from build123d import *

# Parameters (mm, degrees)
F0_W     = 12.7
F0_H     = 25.4
F1_DEPTH = 12.7
F1_TAPER = -3
F2_R     = 7.189125638


with BuildPart() as f1:
    # F0 (on Top) → F1 (new body, symmetric)
    with BuildSketch(Plane.XY):
        with Locations((6.35, 84.2818446611)):
            Rectangle(F0_W, F0_H)
        with Locations((-6.35, 84.2818446611)):
            Rectangle(F0_W, F0_H)
    extrude(amount=F1_DEPTH, both=True, taper=F1_TAPER)

    # F2 (on Front) → F3 (join, up to the next surface of F1)
    with BuildSketch(Plane.XZ):
        Circle(F2_R)
    extrude(until=Until.NEXT, dir=(0, 1, 0))


solid = f1.part
Part model, mm, in its own coordinate system. A direction names the side the tool comes from. Round coordinates to 2 decimals unless told otherwise and drop trailing zeros. Loops run counter-clockwise (first coordinate to the right, second up) from the corner with the lowest first, then second, coordinate; pieces in that order, holes last. Notation, with made-up numbers: (-4, 4) - (44, 4) arc R9 cw to (44, 11) - close; hole circle Ø6 at (85.25, 70.25). An arc over 180 degrees is marked (long way). Answer as a JSON object with one key per item and string values.
Item 1: Tool access for faces 1 (the face through (0, 84, -12.7)), 2 (the face through (-0.936, 35.29, 7.128)): list every direction of +Z, -Z, +X, -X, +Y, -Y with a clear straight run to the whole face (end or side of a thin tool).
Output:
{"face 1": "-Z, +X, -X, +Y, -Y", "face 2": "-Y"}
Item 2: Wall check: L1, parallel to Y at x = -5.5, z = -9.5; L2, parallel to Y at x = -3.5, z = -11; L3, parallel to X at y = 77.5, z = 3. Give the ranges that are in metal, low to high.
Output:
{"L1": "71.08 to 97.48", "L2": "71.01 to 97.56", "L3": "-12.86 to 12.86"}
Item 3: Pin check, flat tips, straight feed: pin 1 (10 mm diameter, centred on x = 1, y = 27.5, fed in from -Z); pin 2 (1 mm diameter, centred on x = 8, y = 14, fed in from +Z); pin 3 (10 mm diameter, centred on y = 68, z = -4, fed in from +X); pin 4 (8 mm diameter, centred on x = -6, z = -7, fed in from +Y). Stop position of each tip, or through.
Output:
{"pin 1": "z = -7.19", "pin 2": "through", "pin 3": "x = 13.11", "pin 4": "y = 97.56"}
Item 4: Band-saw the part on A-A on y = 53. List the corners of the cut face in (x, z), plus the area to 3 significant figures.
Output:
{"outline": "circle Ø14.38 at (0, 0)", "area": "162 mm2"}
